Geometry: final body of the model. Coordinates: model frame, mm. Face numbers are marked on the shaded views. Give positions to 0.01 mm unless a question says otherwise; leave off trailing zeros. Order: outer loops, then holes, each group sorted by start corner. A loop starts at its lowest first (then second) coordinate and runs counter-clockwise, first axis right, second up. Notation, with made-up numbers: (45.5, 23.5) - (96.5, 23.5) arc R12 cw to (96.5, 40.5) - close; hole circle Ø11 at (62, 46.5). An arc over 180 degrees is marked (long way). One line per item, written item: value.
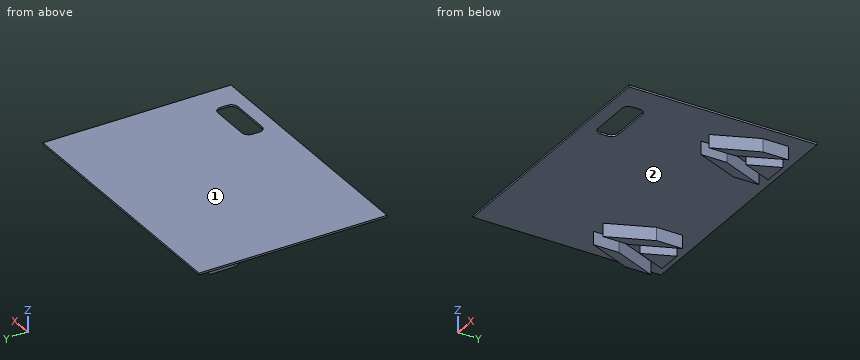
```python
from build123d import *

# Parameters (mm, degrees)
SKETCH1_W           = 97.16644
SKETCH1_H           = 71
SKETCH1_W_2         = 20
SKETCH1_H_2         = 7.62
BOSS_EXTRUDE2_DEPTH = 0.7
BOSS_EXTRUDE3_DEPTH = 5
FILLET1_R           = 2.5


with BuildPart() as part:
    # Sketch1 → Boss-Extrude2 (new body)
    with BuildSketch(Plane.XY):
        with Locations((48.58322, 35.5)):
            Rectangle(SKETCH1_W, SKETCH1_H)
        with Locations((76.731936, 9.000673)):
            Rectangle(SKETCH1_W_2, SKETCH1_H_2, mode=Mode.SUBTRACT)
    extrude(amount=BOSS_EXTRUDE2_DEPTH)

    # Sketch1_4 → Boss-Extrude3 (add)
    with BuildSketch(Plane.XY):
        Polygon((18.516348, 37.85), (18.516348, 47.55), (25.266348, 63.75), (25.266348, 54.05), align=None)
        Polygon((10.891348, 64.75), (20.141348, 64.75), (15.516348, 53.65), align=None)
        Polygon((12.516348, 37.85), (5.766348, 54.05), (5.766348, 63.75), (12.516348, 47.55), align=None)
        Polygon((77.025092, 64.75), (86.275092, 64.75), (81.650092, 53.65), align=None)
        Polygon((79.654973, 47.55), (79.654973, 37.85), (72.904973, 54.05), (72.904973, 63.75), align=None)
        Polygon((84.650092, 37.85), (84.650092, 47.55), (91.400092, 63.75), (91.400092, 54.05), align=None)
    extrude(amount=-BOSS_EXTRUDE3_DEPTH)

    # Fillet1
    fillet1_edges = [part.edges().sort_by_distance(p)[0] for p in [
        (86.731936, 12.810673, 0.35),
        (66.731936, 12.810673, 0.35),
        (66.731936, 5.190673, 0.35),
        (86.731936, 5.190673, 0.35),
    ]]
    fillet(fillet1_edges, radius=FILLET1_R)


solid = part.part
```
1) Material intervals for line 1 along X through (y, z) = (44, -0.6); line 2 along X through (y, z) = (44.5, -0.2); line 3 along X through (y, z) = (61, -4.45), sorted ascending.
Answers below:
line 1: 9.95 to 12.52, 18.52 to 21.08, 77.09 to 79.65, 84.65 to 87.21
line 2: 9.75 to 12.52, 18.52 to 21.29, 76.88 to 79.65, 84.65 to 87.42
line 3: 5.77 to 6.91, 12.45 to 18.58, 24.12 to 25.27, 72.9 to 74.05, 78.59 to 84.71, 90.25 to 91.4
2) Mould query, pull axis X, two halves, no side actions, for the marked faces 1 and 2. Classes: released by +X, released by -X, zero draft, split by the parting line, or undercut.
Answers below:
face 1: zero draft
face 2: undercut
3) First-contact query: pin 1 (1.5 mm diameter, centred on x = 13.5, z = -3.5, fed in from -Y); pin 2 (2.5 mm diameter, centred on x = 83, z = -1.5, fed in from +Y); pin 3 (3 mm diameter, centred on y = 51.5, z = -3, fed in from -X); pin 4 (1 mm diameter, centred on y = 37, z = -3.5, fed in from -X). Flat tips, straight axial feed; report the tip coordinate or a pass-through.
Answers below:
pin 1: y = 56.69
pin 2: y = 64.75
pin 3: x = 6.2
pin 4: through
4) Section B-B, the plane x = 70.5. Return loops of the section in (y, z).
Answers below:
outline: (0, 0) - (5.19, 0) - (5.19, 0.7) - (0, 0.7) - close; (12.81, 0) - (71, 0) - (71, 0.7) - (12.81, 0.7) - close
5) Section D-D, the plane x = 8. Return loops of the section in (y, z).
Answers below:
outline: (0, 0) - (48.69, 0) - (48.69, -5) - (58.39, -5) - (58.39, 0) - (71, 0) - (71, 0.7) - (0, 0.7) - close
6) Section A-A, the plane z = -2.4. Return loops of the section in (x, y), then the cut area to 3 significant figures.
Answers below:
outline: (5.77, 54.05) - (12.52, 37.85) - (12.52, 47.55) - (5.77, 63.75) - close; (10.89, 64.75) - (15.52, 53.65) - (20.14, 64.75) - close; (18.52, 37.85) - (25.27, 54.05) - (25.27, 63.75) - (18.52, 47.55) - close; (72.9, 54.05) - (79.65, 37.85) - (79.65, 47.55) - (72.9, 63.75) - close; (77.03, 64.75) - (81.65, 53.65) - (86.28, 64.75) - close; (84.65, 37.85) - (91.4, 54.05) - (91.4, 63.75) - (84.65, 47.55) - close
area: 365 mm^2
7) Section C-C, the plane y = 55.5. Return loops of the section in (x, z), then the cut area to 3 significant figures.
Answers below:
outline: (0, 0) - (5.77, 0) - (5.77, -5) - (9.2, -5) - (9.2, 0) - (14.75, 0) - (14.75, -5) - (16.29, -5) - (16.29, 0) - (21.83, 0) - (21.83, -5) - (25.27, -5) - (25.27, 0) - (72.9, 0) - (72.9, -5) - (76.34, -5) - (76.34, 0) - (80.88, 0) - (80.88, -5) - (82.42, -5) - (82.42, 0) - (87.96, 0) - (87.96, -5) - (91.4, -5) - (91.4, 0) - (97.17, 0) - (97.17, 0.7) - (0, 0.7) - close
area: 152 mm^2
